The listing builds one solid part. Answer for the finished solid, in the listing's coordinates (mm). A direction names the side the tool comes from. Round coordinates to 2 decimals unless told otherwise and drop trailing zeros. Order: outer loops, then holes, each group sorted by start corner. A loop starts at its lowest first (then second) coordinate and runs counter-clockwise, first axis right, second up. Notation, with made-up numbers: (42.5, 37) -> (79.5, 37) arc R11 ccw to (79.5, 55) -> close; hole circle Ø1 at (35.5, -38.5). An arc over 180 degrees is marked (long way). Return JSON: item names as keys, results as strings. Group by question number.
(1) The part is cut by section B-B (y = 257.5). Determine the outline of the cut face in (x, z).
(2) Each of these flat-tipped pins is pushed along its axis until it touches: pin 1 (4 mm diameter, centred on x = -17.5, z = -96.5, fed in from +Y); pin 2 (16 mm diameter, centred on x = -184, z = -264, fed in from +Y); pin 3 (10 mm diameter, centred on y = 825.5, z = 122, fed in from +X). Where does it stop, or does it pass through?
(3) Consider line 1 (X direction, y = 2.4, z = 264); line 2 (Z direction, x = -184, y = 3.35); line 3 (Z direction, x = -101.5, y = 863). Determine where each line is inside the solid, lowest interval first. Write a range as [from, to].
(4) Which of the six approach directions +Z, -Z, +X, -X, +Y, -Y give full straight-line access (tool end or side, diameter ignored) to faces 5 (the face through (-2, 478, 250)), 6 (the face through (2, 447, -250)), 7 (the face through (170, 547, 3))?
(5) Determine the mould class of faces 1 (the face through (3, 0, 4)), 2 (the face through (-0.91, 822.252, 51.046)), 3 (the face through (62, 906.29, -8.68)), 4 (the face through (-170, 547, -4)) for opening direction Y: +Y half, -Y half, draft (parallel to the pull), parting line (faces both ways), or undercut.
Autodesk Inventor part; units mm, degrees
ref_plane "YZ Plane" through (0, 0, 0) normal (1, 0, 0) x (0, 1, 0)
ref_plane "XZ Plane" through (0, 0, 0) normal (0, 1, 0) x (-1, 0, 0)
ref_plane "XY Plane" through (0, 0, 0) normal (0, 0, 1) x (1, 0, 0)
sketch "Sketch1" plane through (0, 0, 0) normal (0, 1, 0) x (-1, 0, 0)
  line L0 (200, 280) -> (-200, 280)
  line L1 (-200, 280) -> (-200, -280)
  line L2 (-200, -280) -> (200, -280)
  line L3 (200, -280) -> (200, 280)
  line L4 (200, 280) -> (-200, -280) construction
  line L5 (-200, 280) -> (200, -280) construction
  point P0 (0, 0)
extrude "Base" add sketch "Sketch1" along normal blind 5
sketch "Sketch3" plane through (0, 5, 0) normal (0, 1, 0) x (1, 0, 0)
  line L0 (-170, -250) -> (170, -250)
  line L1 (170, -250) -> (170, 250)
  line L2 (170, 250) -> (-170, 250)
  line L3 (-170, 250) -> (-170, -250)
  line L4 (-170, -250) -> (170, 250) construction
  line L5 (170, -250) -> (-170, 250) construction
  point P0 (0, 0)
extrude "Stand" add sketch "Sketch3" along normal blind 900
move faces "Move2" translate (0, 200.25, 0) faces at (56.6667, 905, 83.3333)
chamfer "FrontChamfer" distance 140 angle 25 1 edges at (0, 1105.25, 250) measured on face at (-56.6667, 371.75, 250)
chamfer "BeamHoleFace" distance 202.7 angle 65 1 edges at (0, 1105.25, -250) measured on face at (56.6667, 371.75, -250)
sketch "Sketch5" plane through (-170, 1105.25, 184.6916) normal (0, 0.9063078, -0.4226183) x (1, 0, 0)
  circle A0 centre (170, 239.8145) radius 65
  point P0 (170, 634.4862)
  point P1 (170, 240)
  point P2 (170, 240)
  point P3 (203, 347)
  point P4 (170, 240)
extrude "BeamHole" cut sketch "Sketch5" against normal blind 200
sketch "Sketch6" plane through (0, 5, 0) normal (0, 1, 0) x (1, 0, 0)
  circle A0 centre (-184, -264) radius 5
  circle A1 centre (184, -264) radius 5
  line L0 (200, -280) -> (200, 280) construction
  line L1 (200, 0) -> (-200, 0) construction
  line L2 (-200, 280) -> (-200, -280) construction
  circle A2 centre (-184, 264) radius 5
  circle A3 centre (184, 264) radius 5
  point P0 (0, 0)
extrude "BaseBoltHoles" cut sketch "Sketch6" against normal up to next
properties part number "Base"
Answer below:
{
 "1": {"outline": "(-170, -250) -> (170, -250) -> (170, 250) -> (-170, 250) -> close"},
 "2": {"pin 1": "stops at y = 975.06", "pin 2": "stops at y = 5", "pin 3": "stops at x = 170"},
 "3": {"line 1": "x = [-200, -189], [-179, 179], [189, 200]", "line 2": "z = [-280, -269], [-259, 259], [269, 280]", "line 3": "z = [-250, 250]"},
 "4": {"face 5": "+Z, +X, -X, +Y", "face 6": "-Z, +X, -X, +Y", "face 7": "+Z, -Z, +X, +Y"},
 "5": {"face 1": "-Y half", "face 2": "undercut", "face 3": "undercut", "face 4": "draft"}
}
